from build123d import *

# Parameters (mm, degrees)
SKETCH1_R                                      = 23.401000001
BOSS_EXTRUDE1_DEPTH                            = 2
SKETCH2_R                                      = 1
CUT_EXTRUDE1_DEPTH                             = 10
BOSS_EXTRUDE3_START                            = 1
SKETCH6_R                                      = 1
BOSS_EXTRUDE3_DEPTH                            = 1
CSK_FOR_M3_FLAT_HEAD_MACHINE_SCREW1_AT_2_COUNT = 2
CSK_FOR_M3_FLAT_HEAD_MACHINE_SCREW1_AT_2_PITCH = 53.936


with BuildPart() as part:
    # Sketch1 → Boss-Extrude1 (new body)
    with BuildSketch(Plane(origin=(0, 0, 0), x_dir=(1, 0, 0), z_dir=(0, 1, 0))):
        with BuildLine():
            Line((-103.941978749, -29.858528223), (-100.420009087, -29.669294121))
            Line((-100.420009087, -29.669294121), (-99.403734393, -29.614690064))
            ThreePointArc((-99.403734393, -29.614690064), (-74.666073862, -6.853676168), (-47.63199035, -26.833013765))
            Line((-47.63199035, -26.833013765), (-46.615715656, -26.778409709))
            Line((-46.615715656, -26.778409709), (-43.093745994, -26.589175606))
            Line((-43.093745994, -26.589175606), (-42.55722364, -36.574772421))
            Line((-42.55722364, -36.574772421), (-46.079193302, -36.764006524))
            Line((-46.079193302, -36.764006524), (-47.095467996, -36.81861058))
            ThreePointArc((-47.095467996, -36.81861058), (-71.833128527, -59.579624476), (-98.867212039, -39.60028688))
            Line((-98.867212039, -39.60028688), (-99.883486733, -39.654890936))
            Line((-99.883486733, -39.654890936), (-103.405456395, -39.844125039))
            Line((-103.405456395, -39.844125039), (-103.941978749, -29.858528223))
        make_face()
        with Locations(Location((-73.249601195, -33.216650322, 0), (0, 0, 270))):
            Circle(SKETCH1_R, mode=Mode.SUBTRACT)
    extrude(amount=BOSS_EXTRUDE1_DEPTH)

    # Sketch2 → Cut-Extrude1 (cut)
    with BuildSketch(Plane(origin=(0, 2, 0), x_dir=(1, 0, 0), z_dir=(0, 1, 0))):
        with Locations(Location((-91.776597147, -16.579035648, 0), (0, 0, 270))):
            Circle(SKETCH2_R)
        with Locations(Location((-56.611986521, -14.68965437, 0), (0, 0, 270))):
            Circle(SKETCH2_R)
        with Locations(Location((-54.722605242, -49.854264996, 0), (0, 0, 270))):
            Circle(SKETCH2_R)
        with Locations(Location((-89.887215869, -51.743646275, 0), (0, 0, 270))):
            Circle(SKETCH2_R)
    extrude(amount=-CUT_EXTRUDE1_DEPTH, mode=Mode.SUBTRACT)

    # Sketch6 → Boss-Extrude3 (add)
    # profile 1 of 2: a face of its own
    with BuildSketch(Plane.XZ.offset(BOSS_EXTRUDE3_START)):
        with BuildLine():
            ThreePointArc((-47.095467996, 36.81861058), (-71.833128527, 59.579624476), (-98.867212039, 39.60028688))
            Line((-98.867212039, 39.60028688), (-95.809008422, 39.435970752))
            ThreePointArc((-95.809008422, 39.435970752), (-71.994085233, 56.583945432), (-50.153671613, 36.982926708))
            Line((-50.153671613, 36.982926708), (-47.095467996, 36.81861058))
        make_face()
        with Locations(Location((-89.887215869, 51.743646275, 0), (0, 0, 90))):
            Circle(SKETCH6_R, mode=Mode.SUBTRACT)
        with Locations(Location((-54.722605242, 49.854264996, 0), (0, 0, 90))):
            Circle(SKETCH6_R, mode=Mode.SUBTRACT)
    # profile 2 of 2: a face of its own
    with BuildSketch(Plane.XZ.offset(BOSS_EXTRUDE3_START)):
        with BuildLine():
            ThreePointArc((-50.690193967, 26.997329893), (-74.505117156, 9.849355213), (-96.345530776, 29.450373936))
            Line((-96.345530776, 29.450373936), (-99.403734393, 29.614690064))
            ThreePointArc((-99.403734393, 29.614690064), (-74.666073862, 6.853676168), (-47.63199035, 26.833013765))
            Line((-47.63199035, 26.833013765), (-50.690193967, 26.997329893))
        make_face()
        with Locations(Location((-91.776597147, 16.579035648, 0), (0, 0, 90))):
            Circle(SKETCH6_R, mode=Mode.SUBTRACT)
        with Locations(Location((-56.611986521, 14.68965437, 0), (0, 0, 90))):
            Circle(SKETCH6_R, mode=Mode.SUBTRACT)
    extrude(amount=-BOSS_EXTRUDE3_DEPTH)

    # Sketch9 → CSK for M3 Flat Head Machine Screw1 (revolve, cut)
    with BuildSketch(Plane(origin=(-100.178758687, 2, 34.663543807), x_dir=(0, 0, 1), z_dir=(1, 0, 0))):
        Polygon((0, 0), (0, 3.000025), (1.7, 3.000025), (1.7, 1.45), (3.15, 0), align=None)
    csk_for_m3_flat_head_machine_screw1 = revolve(axis=Axis((-100.178758687, 8.35, 34.663543807), (0, -1, 0)), mode=Mode.SUBTRACT)

    # CSK for M3 Flat Head Machine Screw1 at 2: CSK for M3 Flat Head Machine Screw1 ×2
    with Locations(*[Vector(0.9985596815585082, 0, -0.05365223542193572) * (i * CSK_FOR_M3_FLAT_HEAD_MACHINE_SCREW1_AT_2_PITCH) for i in range(1, CSK_FOR_M3_FLAT_HEAD_MACHINE_SCREW1_AT_2_COUNT)]):
        add(csk_for_m3_flat_head_machine_screw1, mode=Mode.SUBTRACT)


solid = part.part
Design review of the part built by this model. Coordinates are the model's own, in mm. Round coordinates to 2 decimals unless told otherwise and drop trailing zeros. Write each loop counter-clockwise with the first axis right and the second up, starting at its lowest first coordinate (ties: lowest second). Pieces come first, ordered by that corner, then holes. Notation, with made-up numbers: (77, -28) -> (119, -28) arc R10 cw to (119, -22) -> close; hole circle Ø7 at (-13, -36). An arc over 180 degrees is marked (long way). One line per item, written item: value. Start each with the question number.
Q1. The part is to be moulded in two halves that separate along X. For faces 1 (the face through (-103.67, 0.99, 34.92)), 2 (the face through (-90.88, 0.48, 51.61)), 3 (the face through (-69, -1, 57)), 4 (the face through (-53.835, 0.479, 50.316)), say which applies: pulls with the +X half, pulls with the -X half, needs draft (parallel to the pull), parting line crosses it, or undercut.
Q2. Add section C-C (y = 1.1). Give the boundary of the cut face in (x, z).
Q3. To check wall thickness, follow probe 1 along Z at (x, y) = (-72.5, 1.35); probe 2 along Z at (x, y) = (-56.5, 1.3); probe 3 along Z at (x, y) = (-92.5, 0.6). State the ranges of each line that lie inside material, in increasing order.
Q4. Add section B-B (z = 55.5). Give the boundary of the cut face in (x, y), then the cut area to 3 significant figures.
Q5. Insertion check: P1, Ø4, axis at x = -46.32, z = 31.77, coming from the -Y side; P2, Ø1, axis at x = -79, y = 0, coming from the -Z side; P3, Ø1.6, axis at x = -54.72, z = 49.85, coming from the -Y side (3 decimals); P4, Ø2.5, axis at x = -56.61, z = 14.69, coming from the +Y side. Each pin has a flat end and moves straight along its axis. Give the tip position at first contact, or say it passes through.
Q6. Add section A-A (x = -68.5). Give the boundary of the cut face in (y, z), then the cut area to 3 significant figures.
Response:
1. face 1: pulls with the -X half
1. face 2: undercut
1. face 3: needs draft
1. face 4: undercut
2. outline: (-103.94, 29.86) -> (-99.4, 29.61) arc R26.4 ccw to (-47.63, 26.83) -> (-43.09, 26.59) -> (-42.56, 36.57) -> (-47.1, 36.82) arc R26.4 ccw to (-98.87, 39.6) -> (-103.41, 39.84) -> close; hole circle Ø4.5 at (-100.18, 34.66); hole circle Ø46.8 at (-73.25, 33.22); hole circle Ø2 at (-91.78, 16.58); hole circle Ø2 at (-89.89, 51.74); hole circle Ø2 at (-56.61, 14.69); hole circle Ø2 at (-54.72, 49.85); hole circle Ø4.5 at (-46.32, 31.77)
3. probe 1: z = 6.83 to 9.83, 56.61 to 59.61
3. probe 2: z = 12.81 to 13.7, 15.68 to 16.87, 49.56 to 53.62
3. probe 3: z = 15.15 to 15.89, 17.27 to 19.91, 46.52 to 51.28
4. outline: (-87.41, -1) -> (-80.4, -1) -> (-80.4, 2) -> (-87.41, 2) -> close; (-66.1, -1) -> (-59.09, -1) -> (-59.09, 2) -> (-66.1, 2) -> close
4. area: 42.1 mm^2
5. P1: stops at y = 0
5. P2: stops at z = 7.34
5. P3: passes through
5. P4: stops at y = 2
6. outline: (-1, 7.25) -> (2, 7.25) -> (2, 10.3) -> (-1, 10.3) -> close; (-1, 56.13) -> (2, 56.13) -> (2, 59.19) -> (-1, 59.19) -> close
6. area: 18.3 mm^2
